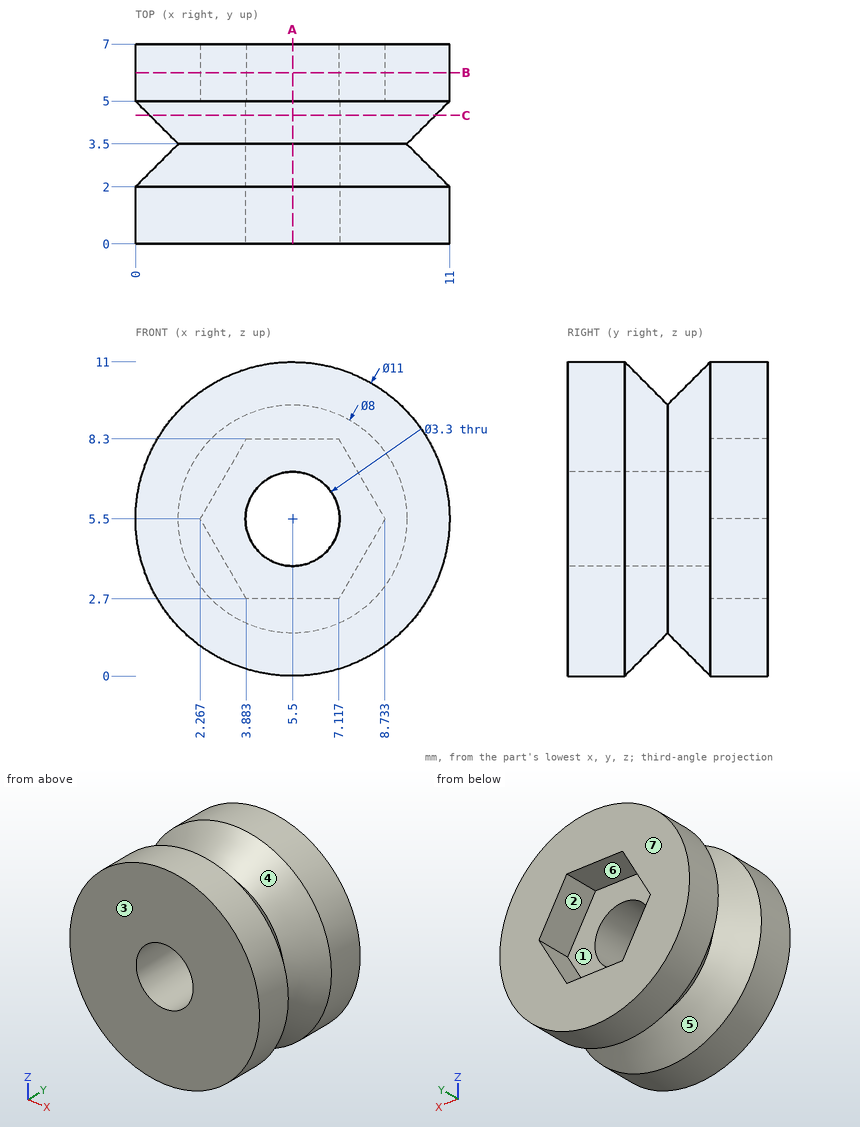
Could you check a few things on this drawing? It's one solid part, dimensions in mm from its lowest x, y, z. A direction names the side the tool comes from. Round coordinates to 2 decimals unless told otherwise and drop trailing zeros. Loops run counter-clockwise (first coordinate to the right, second up) from the corner with the lowest first, then second, coordinate; pieces in that order, holes last.
Q1. Please list where these lines run through material, in increasing order: L1, parallel to Z at x = 5.5, y = 1.5; L2, parallel to Y at x = 5.75, z = 8.
Q2. I want a section at B-B (y = 6). Write out the boundary of the cut face in (x, z).
Q3. For P1, Ø1.7, axis at x = 6.5, z = 6.5, coming from the +Y side; P2, Ø4, axis at x = 2.5, y = 5.5, coming from the +Z side; P3, Ø2, axis at x = 3.5, y = 3.5, coming from the +Z side (1 decimal), each with a flat end and sliding along its axis, tell me the tip position at first contact or that it passes through.
Q4. I want a section at C-C (y = 4.5). Write out the boundary of the cut face in (x, z), and give its area (3 significant figures).
Q5. On a 3-axis mill with a long thin cutter (end or side, diameter ignored), from which of +Z, -Z, +X, -X, +Y, -Y can I reach the whole of each face in a straight line? I mean the marked faces 5, 6 and 7. Say none if no direction works.
Q6. Thinking about a two-plate mould opening in Z: for the marked faces 1, 2, 3 and 4, which applies, pulls with the +Z half, pulls with the -Z half, needs draft (parallel to the pull), parting line crosses it, or undercut?
Q7. I want a section at A-A (x = 5.5). Write out the boundary of the cut face in (y, z), and give its area (3 significant figures).
Answer below:
1. L1: z = 0 to 3.85, 7.15 to 11
1. L2: y = 0 to 5
2. outline: circle Ø11 at (5.5, 5.5); hole (2.27, 5.5) - (3.88, 2.7) - (7.12, 2.7) - (8.73, 5.5) - (7.12, 8.3) - (3.88, 8.3) - close
3. P1: stops at y = 5
3. P2: stops at z = 10.91
3. P3: stops at z = 10.2
4. outline: circle Ø10 at (5.5, 5.5); hole circle Ø3.3 at (5.5, 5.5)
4. area: 70.0 mm2
5. face 5: none
5. face 6: +Y
5. face 7: +Z, -Z, +X, -X, +Y
6. face 1: undercut
6. face 2: undercut
6. face 3: needs draft
6. face 4: parting line crosses it
7. outline: (0, 0) - (2, 0) - (3.5, 1.5) - (5, 0) - (7, 0) - (7, 2.7) - (5, 2.7) - (5, 3.85) - (0, 3.85) - close; (0, 7.15) - (5, 7.15) - (5, 8.3) - (7, 8.3) - (7, 11) - (5, 11) - (3.5, 9.5) - (2, 11) - (0, 11) - close
7. area: 44.8 mm2
